Work out the finished part from the listing and answer in its coordinate system (mm). Face numbers are marked on the shaded views. A direction names the side the tool comes from. Round coordinates to 2 decimals unless told otherwise and drop trailing zeros. Write each loop counter-clockwise with the first axis right and the second up, starting at its lowest first coordinate (ties: lowest second). Pieces come first, ordered by that corner, then holes.
1. Straight lines are drawn through the part: probe 1 along Z at (x, y) = (21, 6); probe 2 along X at (y, z) = (29.5, 6.5); probe 3 along Y at (x, z) = (-9.5, -29). For each, find the intervals that lie inside material, in ascending order.
2. A tool of negligible diameter and unlimited length cuts with its end or side. For the marked faces 1, 2, 3 and 4, from which of +Z, -Z, +X, -X, +Y, -Y can it reach the whole face along a straight path? Write none if from no direction.
3. Find section D-D (y = 32.5). Write down the section's boundary in (x, z), and give its area (3 significant figures).
4. Find section C-C (x = -5.5). Write down the section's boundary in (y, z), and give its area (3 significant figures).
5. Find section A-A (y = 19). Write down the section's boundary in (x, z), and give its area (3 significant figures).
6. Flat-ended cylindrical pins translate along their axes: pin 1 Ø5 at (x, y) = (19.5, 21) entering from +Z; pin 2 Ø11.5 at (y, z) = (18.5, 2.5) entering from +X; pin 3 Ø3 at (x, z) = (-16.5, -13) entering from -Y. Find the tip coordinate at first contact, or state that the pin passes through.
7. Find section B-B (z = -24). Write down the section's boundary in (x, y), and give its area (3 significant figures).
```python
from build123d import *

# Parameters (mm, degrees)
F1_DEPTH = 38
F2_W     = 8
F2_H     = 40
F3_DEPTH = 43.3
F5_DEPTH = 11
F7_DEPTH = 11
F9_DEPTH = 42.4


with BuildPart() as f1:
    # F0 (on Front) → F1 (new body)
    with BuildSketch(Plane.XZ):
        Polygon((-20.403226763, 14.420258379), (-31.403226763, 14.420258379), (-31.403226763, -42.579741621), (25.596773237, -42.579741621), (25.596773237, -31.579741621), (-20.403226763, -31.579741621), align=None)
    extrude(amount=-F1_DEPTH)

    # F2 (on face) → F3 (join)
    with BuildSketch(Plane.YZ.offset(-20.403226763)):
        Polygon((23, -31.579741621), (15, -31.579741621), (26, -37.2273437679), (34.1856418401, -37.2273437679), align=None)
        with Locations((19, -11.579741621)):
            Rectangle(F2_W, F2_H)
    extrude(amount=F3_DEPTH)

    # F4 (on face) → F5 (join)
    with BuildSketch(Plane.XY.offset(-31.579741621)):
        with BuildLine():
            Line((25.596773237, 38), (25.596773237, 0))
            ThreePointArc((25.596773237, 0), (40.596773237, 19), (25.596773237, 38))
        make_face()
    extrude(amount=-F5_DEPTH)

    # F6 (on face) → F7 (join)
    with BuildSketch(Plane.YZ.offset(-20.403226763)):
        with BuildLine():
            Line((0, 14.420258379), (38, 14.420258379))
            ThreePointArc((38, 14.420258379), (19, 34.420258379), (0, 14.420258379))
        make_face()
    extrude(amount=-F7_DEPTH)

    # F8 (on face) → F9 (cut)
    with BuildSketch(Plane.XZ.offset(-15)):
        Polygon((22.896773237, 8.420258379), (-20.403226763, 8.420258379), (22.896773237, -31.579741621), align=None)
    extrude(amount=-F9_DEPTH, mode=Mode.SUBTRACT)


solid = f1.part
```
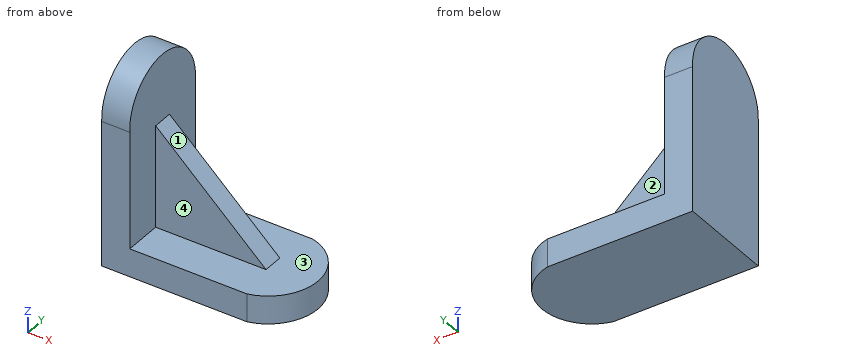
Worked answers:
1. probe 1: z = -42.58 to -31.58
1. probe 2: x = -31.4 to -20.4
1. probe 3: y = 15 to 23
2. face 1: +Z, +X, +Y, -Y
2. face 2: +Z, +X, +Y
2. face 3: +Z, +X
2. face 4: +Z, +X, -Y
3. outline: (-31.4, -42.58) - (35.18, -42.58) - (35.18, -31.58) - (-20.4, -31.58) - (-20.4, 28.8) - (-31.4, 28.8) - close
3. area: 1,400 mm2
4. outline: (0, -42.58) - (38, -42.58) - (38, -31.58) - (23, -31.58) - (23, -5.35) - (15, -5.35) - (15, -31.58) - (0, -31.58) - close
4. area: 628 mm2
5. outline: (-31.4, -42.58) - (40.6, -42.58) - (40.6, -31.58) - (22.9, -31.58) - (-20.4, 8.42) - (-20.4, 34.42) - (-31.4, 34.42) - close
5. area: 2,380 mm2
6. pin 1: stops at z = -26.13
6. pin 2: stops at x = -7.77
6. pin 3: stops at y = 15
7. outline: (-31.4, 0) - (-20.4, 0) - (-20.4, 15) - (14.69, 15) - (14.69, 23) - (-20.4, 23) - (-20.4, 38) - (-31.4, 38) - close
7. area: 699 mm2
